The figure shows three views and two pictorial views of one solid part (mm, origin at its lowest corner). Answer the questions. A direction names the side the tool comes from. Round coordinates to 2 decimals unless told otherwise and drop trailing zeros. Order: outer loops, then holes, each group sorted by start corner. A loop starts at its lowest first (then second) coordinate and runs counter-clockwise, first axis right, second up. Notation, with made-up numbers: (79, 19.25) -> (91, 19.25) arc R19 cw to (91, 54.25) -> close; hole circle Ø11 at (46.25, 29.25). An arc over 180 degrees is marked (long way). One line per item, written item: value. Start each with the question number.
1. Section B-B (y = 0.7) is taken. Give the vertices of the cut face in (x, z), then the cut area to 3 significant figures.
2. Flat-ended cylindrical pins translate along their axes: pin 1 Ø1.8 at (x, z) = (100, 69) entering from +Y; pin 2 Ø1 at (y, z) = (0.5, 8.5) entering from +X; pin 3 Ø2 at (y, z) = (2, 42) entering from +X. Find the tip coordinate at first contact, or state that the pin passes through.
3. Consider line 1 (Z direction, x = 186, y = 2.1); line 2 (X direction, y = 3.3, z = 11); line 3 (X direction, y = 1.2, z = 40). Determine where each line is inside the solid, lowest interval first.
4. Section C-C (x = 7.5) is taken. Give the vertices of the cut face in (y, z).
5. Section D-D (z = 29.5) is taken. Give the vertices of the cut face in (x, y), then the cut area to 3 significant figures.
6. Section A-A (x = 158) is taken. Give the vertices of the cut face in (y, z), then the cut area to 3 significant figures.
7. For the marked faces 1 and 2, determine the directions among +Z, -Z, +X, -X, +Y, -Y from which every point of the face is accessible in a straight line to the end or side of a thin tool.
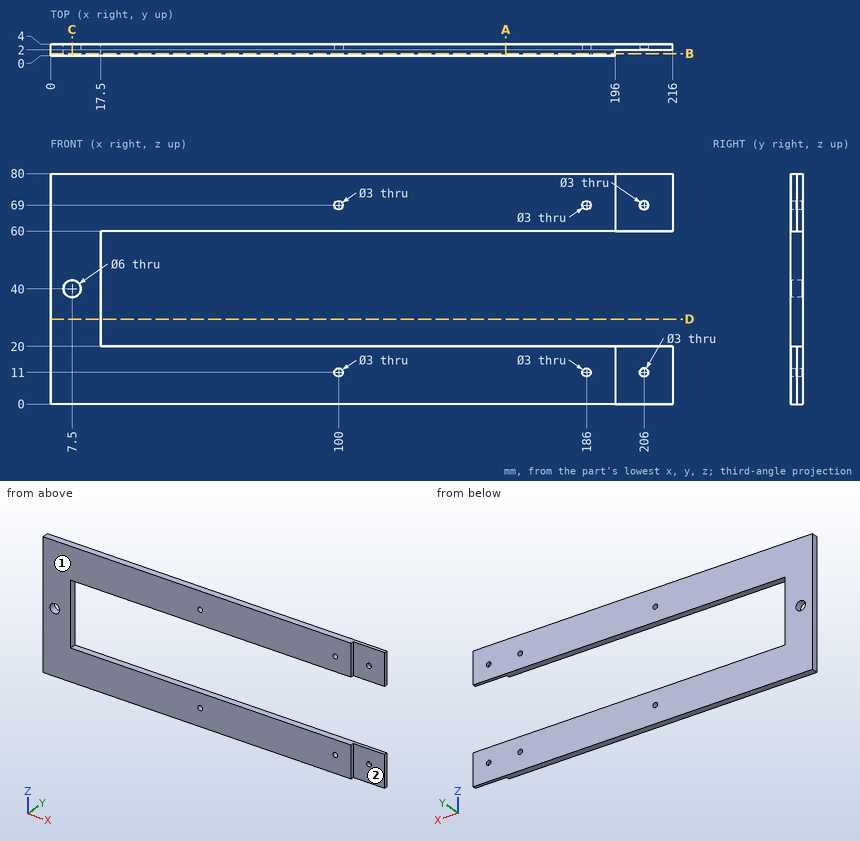
Answer:
1. outline: (0, 0) -> (196, 0) -> (196, 20) -> (17.5, 20) -> (17.5, 60) -> (196, 60) -> (196, 80) -> (0, 80) -> close; hole circle Ø6 at (7.5, 40); hole circle Ø3 at (100, 11); hole circle Ø3 at (100, 69); hole circle Ø3 at (186, 11); hole circle Ø3 at (186, 69)
1. area: 8,480 mm^2
2. pin 1: through
2. pin 2: x = 196
2. pin 3: x = 17.5
3. line 1: 0 to 9.5, 12.5 to 20, 60 to 67.5, 70.5 to 80
3. line 2: 0 to 98.5, 101.5 to 184.5, 187.5 to 204.5, 207.5 to 216
3. line 3: 0 to 4.5, 10.5 to 17.5
4. outline: (0, 0) -> (4, 0) -> (4, 37) -> (0, 37) -> close; (0, 43) -> (4, 43) -> (4, 80) -> (0, 80) -> close
5. outline: (0, 0) -> (17.5, 0) -> (17.5, 4) -> (0, 4) -> close
5. area: 70.0 mm^2
6. outline: (0, 0) -> (4, 0) -> (4, 20) -> (0, 20) -> close; (0, 60) -> (4, 60) -> (4, 80) -> (0, 80) -> close
6. area: 160 mm^2
7. face 1: +Z, -Z, +X, -X, -Y
7. face 2: +Z, -Z, +X, -Y
